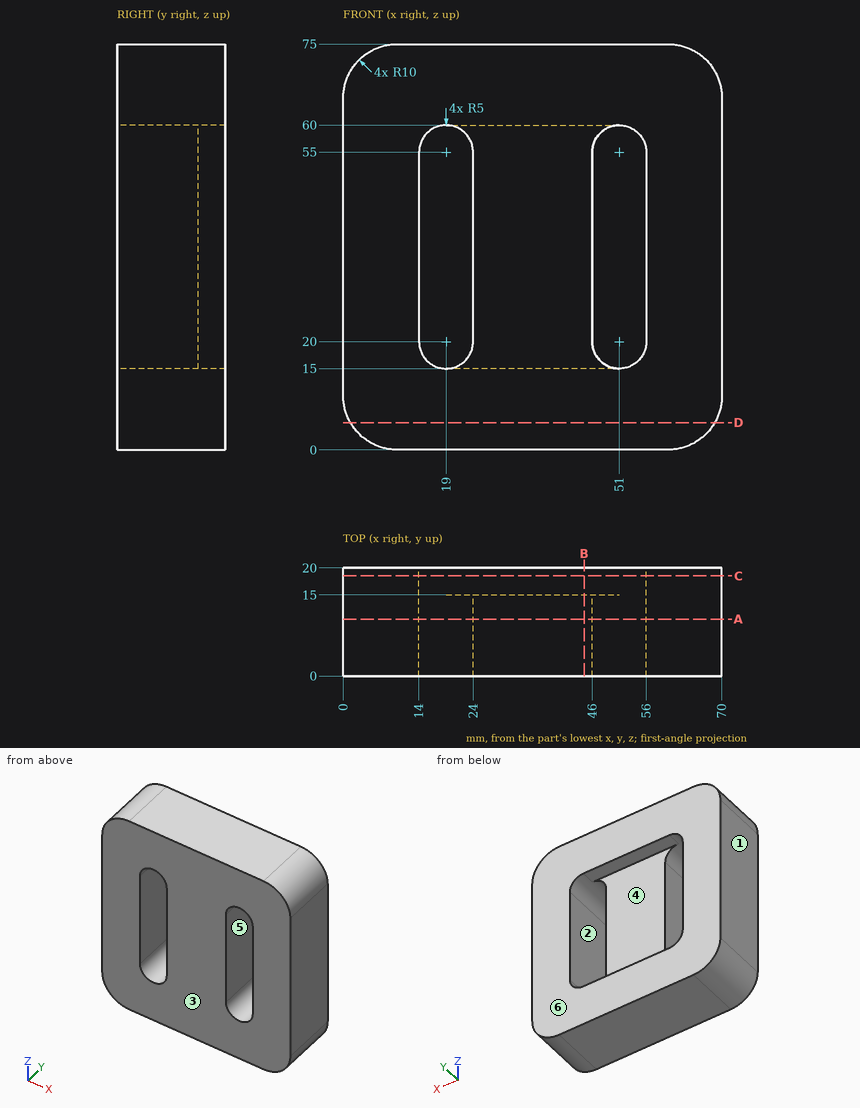
Can you work these out from the drawing? Everything is in mm from the part's minimum corner. A direction names the side the tool comes from. Round coordinates to 2 decimals unless told otherwise and drop trailing zeros. Write each loop counter-clockwise with the first axis right and the second up, starting at its lowest first coordinate (ties: lowest second). Pieces come first, ordered by that corner, then holes. Notation, with made-up numbers: (53.25, -6) - (106.25, -6) arc R14 cw to (106.25, 17) - close; hole circle Ø8 at (69, -14). An arc over 180 degrees is marked (long way). Put each result on its own line as item: value. Start each with the question number.
(1) I want a section at B-B, the plane x = 44.5. Please give me the cut outline in (y, z), plus the area to 4 significant figures.
(2) I want a section at C-C, the plane y = 18.5. Please give me the cut outline in (x, z).
(3) I want a section at D-D, the plane z = 5. Please give me the cut outline in (x, y), plus the area to 3 significant figures.
(4) I want a section at A-A, the plane y = 10.5. Please give me the cut outline in (x, z).
(5) Thinking about a two-plate mould opening in X: for the marked faces 1, 2 and 3, which applies, released by +X, released by -X, zero draft, split by the parting line, or undercut?
(6) For the marked faces 4, 5 and 6, which set-ups out of +Z, -Z, +X, -X, +Y, -Y let a thin tool reach every point of the face, with its end or its side?
(7) I need wall thicknesses on probe 1 along X at (y, z) = (8.25, 43); probe 2 along X at (y, z) = (15.5, 38); probe 3 along X at (y, z) = (13.25, 56). Which ranges of each line are inside material? Lowest first, please.
Here are the results:
1. outline: (0, 0) - (20, 0) - (20, 15) - (15, 15) - (15, 60) - (20, 60) - (20, 75) - (0, 75) - close
1. area: 1,275 mm^2
2. outline: (0, 10) arc R10 ccw to (10, 0) - (60, 0) arc R10 ccw to (70, 10) - (70, 65) arc R10 ccw to (60, 75) - (10, 75) arc R10 ccw to (0, 65) - close; hole (14, 20) arc R5 ccw to (19, 15) - (51, 15) arc R5 ccw to (56, 20) - (56, 55) arc R5 ccw to (51, 60) - (19, 60) arc R5 ccw to (14, 55) - close
3. outline: (1.34, 0) - (68.66, 0) - (68.66, 20) - (1.34, 20) - close
3. area: 1,350 mm^2
4. outline: (0, 10) arc R10 ccw to (10, 0) - (60, 0) arc R10 ccw to (70, 10) - (70, 65) arc R10 ccw to (60, 75) - (10, 75) arc R10 ccw to (0, 65) - close; hole (14, 20) arc R5 ccw to (24, 20) - (24, 55) arc R5 ccw to (14, 55) - close; hole (46, 20) arc R5 ccw to (56, 20) - (56, 55) arc R5 ccw to (46, 55) - close
5. face 1: released by -X
5. face 2: undercut
5. face 3: zero draft
6. face 4: +Y
6. face 5: +Y, -Y
6. face 6: +Z, -Z, +X, -X, +Y
7. probe 1: x = 0 to 14, 24 to 46, 56 to 70
7. probe 2: x = 0 to 14, 56 to 70
7. probe 3: x = 0 to 14.1, 23.9 to 46.1, 55.9 to 70
